from build123d import *

# Parameters (mm, degrees)
BOSS_EXTRUDE1_DEPTH     = 3
SKETCH2_W               = 5
SKETCH2_H               = 3
CUT_EXTRUDE1_DEPTH      = 45.699303997
SKETCH3_W               = 18.054262684
SKETCH3_H               = 80.34146894
BOSS_EXTRUDE2_DEPTH     = 5
SKETCH5_W               = 11.91581337
SKETCH5_H               = 76.008445896
CUT_EXTRUDE2_DEPTH      = 5
CUT_EXTRUDE3_DEPTH      = 45.877920827
CUT_EXTRUDE3_DEPTH_BACK = 45.877920827
SKETCH7_W               = 2
SKETCH7_H               = 9
BOSS_EXTRUDE3_DEPTH     = 5
CUT_EXTRUDE4_DEPTH      = 5
SKETCH9_W               = 2.534423144
SKETCH9_H               = 2
CUT_EXTRUDE5_DEPTH      = 1
CUT_EXTRUDE6_DEPTH      = 2
BOSS_EXTRUDE5_DEPTH     = 2
BOSS_EXTRUDE6_DEPTH     = 2
CUT_EXTRUDE7_START      = -2
CUT_EXTRUDE7_DEPTH      = 2


with BuildPart() as part:
    # Sketch1 → Boss-Extrude1 (new body)
    with BuildSketch(Plane(origin=(0, 0, 0), x_dir=(0, 0, -1), z_dir=(1, 0, 0))):
        with BuildLine():
            Line((-8.833333333, -43), (11.833333333, -43))
            Line((11.833333333, -43), (11.833333333, 43))
            Line((11.833333333, 43), (-8.833333333, 43))
            ThreePointArc((-8.833333333, 43), (-10.954653677, 42.121320344), (-11.833333333, 40))
            Line((-11.833333333, 40), (-11.833333333, -40))
            ThreePointArc((-11.833333333, -40), (-10.954653677, -42.121320344), (-8.833333333, -43))
        make_face()
    extrude(amount=BOSS_EXTRUDE1_DEPTH)

    # Sketch2 → Cut-Extrude1 (cut, through all)
    with BuildSketch(Plane(origin=(3, 0, 0), x_dir=(0, 0, -1), z_dir=(1, 0, 0))):
        with Locations((0, -34.060962647)):
            Rectangle(SKETCH2_W, SKETCH2_H)
    extrude(amount=-CUT_EXTRUDE1_DEPTH, mode=Mode.SUBTRACT)

    # Sketch3 → Boss-Extrude2 (add)
    with BuildSketch(Plane.ZY):
        Rectangle(SKETCH3_W, SKETCH3_H)
    extrude(amount=BOSS_EXTRUDE2_DEPTH)

    # Sketch5 → Cut-Extrude2 (cut)
    with BuildSketch(Plane.ZY.offset(5)):
        Rectangle(SKETCH5_W, SKETCH5_H)
    extrude(amount=-CUT_EXTRUDE2_DEPTH, mode=Mode.SUBTRACT)

    # Sketch6 → Cut-Extrude3 (cut, two sides: drawn at the far end of the back side and taken through both)
    with BuildSketch(Plane.XY.offset(-CUT_EXTRUDE3_DEPTH_BACK)):
        Polygon((-5, -19.974207963), (-1.714874455, -16.689082418), (-1.714874455, 16.689082418), (-5, 19.974207963), align=None)
    extrude(amount=CUT_EXTRUDE3_DEPTH + CUT_EXTRUDE3_DEPTH_BACK, mode=Mode.SUBTRACT)

    # Sketch7 → Boss-Extrude3 (add)
    with BuildSketch(Plane.ZY):
        Rectangle(SKETCH7_W, SKETCH7_H)
    extrude(amount=BOSS_EXTRUDE3_DEPTH)

    # Sketch8 → Cut-Extrude4 (cut)
    with BuildSketch(Plane.XY.offset(1)):
        with BuildLine():
            ThreePointArc((-5, -0.459578833), (-2.44210099, -2.530530169), (0, -0.32421434))
            Line((0, -0.32421434), (0, 0.32421434))
            ThreePointArc((0, 0.32421434), (-2.44210099, 2.530530169), (-5, 0.459578833))
            Line((-5, 0.459578833), (-5, -0.459578833))
        make_face()
        with BuildLine():
            Line((-5, -4.5), (-2.510609776, -4.5))
            ThreePointArc((-2.510609776, -4.5), (-3.81075192, -4.308088951), (-5, -3.748724625))
            Line((-5, -3.748724625), (-5, -4.5))
        make_face()
        with BuildLine():
            Line((-2.510609776, -4.5), (0, -4.5))
            Line((0, -4.5), (0, -3.734546632))
            ThreePointArc((0, -3.734546632), (-1.198256898, -4.304384965), (-2.510609776, -4.5))
        make_face()
        with BuildLine():
            ThreePointArc((-2.510609794, 4.5), (-1.198256907, 4.304384967), (0, 3.734546632))
            Line((0, 3.734546632), (0, 4.5))
            Line((0, 4.5), (-2.510609794, 4.5))
        make_face()
        with BuildLine():
            ThreePointArc((-5, 3.748724625), (-3.810751929, 4.308088948), (-2.510609794, 4.5))
            Line((-2.510609794, 4.5), (-5, 4.5))
            Line((-5, 4.5), (-5, 3.748724625))
        make_face()
    extrude(amount=-CUT_EXTRUDE4_DEPTH, mode=Mode.SUBTRACT)

    # Sketch9 → Cut-Extrude5 (cut)
    with BuildSketch(Plane.ZY.offset(5)):
        Rectangle(SKETCH9_W, SKETCH9_H)
    extrude(amount=-CUT_EXTRUDE5_DEPTH, mode=Mode.SUBTRACT)

    # Sketch12 → Cut-Extrude6 (cut)
    with BuildSketch(Plane.XY.offset(1)):
        with BuildLine():
            Line((-4.836179898, -1), (-5, -1))
            Line((-5, -1), (-5, -3.748724625))
            ThreePointArc((-5, -3.748724625), (-2.497849634, -4.499981909), (0, -3.734546632))
            Line((0, -3.734546632), (0, -0.32421434))
            ThreePointArc((0, -0.32421434), (-2.160279243, -2.507098902), (-4.836179898, -1))
        make_face()
        with BuildLine():
            Line((-5, 3.748724625), (-5, 1))
            Line((-5, 1), (-4.836179898, 1))
            ThreePointArc((-4.836179898, 1), (-2.160279243, 2.507098902), (0, 0.32421434))
            Line((0, 0.32421434), (0, 3.734546632))
            ThreePointArc((0, 3.734546632), (-2.497849634, 4.499981909), (-5, 3.748724625))
        make_face()
    extrude(amount=-CUT_EXTRUDE6_DEPTH, mode=Mode.SUBTRACT)

    # Sketch10 → Boss-Extrude5 (add)
    with BuildSketch(Plane.XY.offset(1)):
        with BuildLine():
            Line((0.632034053, -1.144834058), (-0.193, -4.453864907))
            ThreePointArc((-0.193, -4.453864907), (-2.801828378, -4.592278965), (-5.047908598, -3.258012274))
            Line((-5.047908598, -3.258012274), (-4.41989103, -0.739171385))
            Line((-4.41989103, -0.739171385), (-4.335953587, -0.66680401))
            ThreePointArc((-4.335953587, -0.66680401), (-2.053682052, -3.002243354), (0.632034053, -1.144834058))
        make_face()
        with BuildLine():
            Line((-5.047908598, 3.258012274), (-4.41989103, 0.739171385))
            Line((-4.41989103, 0.739171385), (-4.335953587, 0.66680401))
            ThreePointArc((-4.335953587, 0.66680401), (-2.053682052, 3.002243354), (0.632034053, 1.144834058))
            Line((0.632034053, 1.144834058), (-0.193, 4.453864907))
            ThreePointArc((-0.193, 4.453864907), (-2.801828378, 4.592278965), (-5.047908598, 3.258012274))
        make_face()
    extrude(amount=-BOSS_EXTRUDE5_DEPTH)

    # Sketch13 → Boss-Extrude6 (add)
    with BuildSketch(Plane(origin=(0, 0, -1), x_dir=(-1, 0, 0), z_dir=(0, 0, -1))):
        Polygon((0, 3.679784186), (0.193, 4.453864907), (-0.617433114, 4.244828064), (-0.739085506, -4.079345447), (0.193, -4.453864907), (0, -3.679784186), (0, -2.250971384), (0, 2.250971384), align=None)
    extrude(amount=-BOSS_EXTRUDE6_DEPTH)

    # Sketch15 → Cut-Extrude7 (cut)
    with BuildSketch(Plane(origin=(0, 0, -1), x_dir=(-1, 0, 0), z_dir=(0, 0, -1)).offset(CUT_EXTRUDE7_START)):
        Polygon((4.65583066, 1.685473556), (5.047908598, 3.258012274), (4.038538563, 1.685473556), align=None)
        with BuildLine():
            Line((4.65583066, 1.685473556), (4.038538563, 1.685473556))
            ThreePointArc((4.038538563, 1.685473556), (4.241224486, 1.191898546), (4.335953587, 0.66680401))
            Line((4.335953587, 0.66680401), (4.41989103, 0.739171385))
            Line((4.41989103, 0.739171385), (4.65583066, 1.685473556))
        make_face()
        with BuildLine():
            ThreePointArc((4.335953587, -0.66680401), (4.241224486, -1.191898546), (4.038538563, -1.685473556))
            Line((4.038538563, -1.685473556), (4.65583066, -1.685473556))
            Line((4.65583066, -1.685473556), (4.41989103, -0.739171385))
            Line((4.41989103, -0.739171385), (4.335953587, -0.66680401))
        make_face()
        Polygon((4.65583066, -1.685473556), (4.038538563, -1.685473556), (5.047908598, -3.258012274), align=None)
    extrude(amount=CUT_EXTRUDE7_DEPTH, mode=Mode.SUBTRACT)


solid = part.part
Source: CAD feature listing. Evaluate the final solid. Frame: model axes, mm. A direction names the side the tool comes from. Give positions to 0.01 mm unless a question says otherwise; leave off trailing zeros. Write each loop counter-clockwise with the first axis right and the second up, starting at its lowest first coordinate (ties: lowest second). Pieces come first, ordered by that corner, then holes. Notation, with made-up numbers: (-26, -4.5) -> (2, -4.5) arc R25 ccw to (2, 34.5) -> close; hole circle Ø3 at (24.25, 86). An arc over 180 degrees is marked (long way). Return JSON: item names as keys, results as strings. Group by question number.
1. Section B-B, the plane y = 10.5. Output: boundary loops of the cut face in (x, z).
2. Pin query (flat end, axial travel): pin 1 Ø10 at (y, z) = (10.5, -1) entering from -X; pin 2 Ø2.5 at (x, y) = (-3.5, -15) entering from -Z; pin 3 Ø5 at (y, z) = (-17, -9) entering from -X; pin 4 Ø1.5 at (x, z) = (-2.5, -1.5) entering from -Y. Return the tip coordinate at first contact, or that it passes through.
3. Section A-A, the plane z = 1.75. Output: boundary loops of the cut face in (x, y), then the cut area to 3 significant figures.
4. Section C-C, the plane x = -3. Output: boundary loops of the cut face in (y, z), then the cut area to 3 significant figures.
5. Mould query, pull axis Z, two halves, no side actions, for faces 1 (the face through (-1.715, 0, -8)), 2 (the face through (1.479, -42.098, 10.978)), 3 (the face through (-2.195, 2.985, 0.014)). Classes: +Z half, -Z half, draft (parallel to the pull), parting line (faces both ways), or undercut.
6. Access query for faces 4 (the face through (-3, 38.004, 0)), 5 (the face through (-3.334, 18.309, 7.471)), 6 (the face through (-2, -40.171, 0)). Directions: +Z, -Z, +X, -X, +Y, -Y. A direction counts if a zero-diameter tool reaches every point of the face in a straight line with its end or side. Return the directions, or none.
7. Material intervals for line 1 (Y direction, x = -1.75, z = -2.75); line 2 (Z direction, x = -2.5, y = 34); line 3 (X direction, y = 1, z = -6), sorted ascending. Write a range as from..to.
8. Section D-D, the plane z = -8.25. Output: boundary loops of the cut face in (x, y).
Determined:
{
 "1": {"outline": "(-1.71, -9.03) -> (0, -9.03) -> (0, -11.83) -> (3, -11.83) -> (3, 11.83) -> (0, 11.83) -> (0, 9.03) -> (-1.71, 9.03) -> (-1.71, 5.96) -> (0, 5.96) -> (0, -5.96) -> (-1.71, -5.96) -> close"},
 "2": {"pin 1": "stops at x = -1.71", "pin 2": "passes through", "pin 3": "stops at x = -4.53", "pin 4": "stops at y = -40.17"},
 "3": {"outline": "(-5, -40.17) -> (0, -40.17) -> (0, -43) -> (3, -43) -> (3, -35.56) -> (0, -35.56) -> (0, -38) -> (-5, -38) -> close; (-5, 38) -> (0, 38) -> (0, -32.56) -> (3, -32.56) -> (3, 43) -> (0, 43) -> (0, 40.17) -> (-5, 40.17) -> close", "area": "271 mm2"},
 "4": {"outline": "(-40.17, -9.03) -> (-17.97, -9.03) -> (-17.97, -5.96) -> (-38, -5.96) -> (-38, 5.96) -> (-17.97, 5.96) -> (-17.97, 9.03) -> (-40.17, 9.03) -> close; (-4.54, -1) -> (-2.72, -1) -> (-2.72, 1) -> (-4.54, 1) -> close; (2.72, -1) -> (4.54, -1) -> (4.54, 1) -> (2.72, 1) -> close; (17.97, -9.03) -> (40.17, -9.03) -> (40.17, 9.03) -> (17.97, 9.03) -> (17.97, 5.96) -> (38, 5.96) -> (38, -5.96) -> (17.97, -5.96) -> close", "area": "331 mm2"},
 "5": {"face 1": "draft", "face 2": "+Z half", "face 3": "undercut"},
 "6": {"face 4": "-X", "face 5": "+Z, -Z, -X", "face 6": "+Z, -Z, -X, -Y"},
 "7": {"line 1": "y = -40.17..-38, 38..40.17", "line 2": "z = -9.03..-5.96, 5.96..9.03", "line 3": "x = -1.71..3"},
 "8": {"outline": "(-5, -40.17) -> (0, -40.17) -> (0, -43) -> (3, -43) -> (3, 43) -> (0, 43) -> (0, 40.17) -> (-5, 40.17) -> (-5, 19.97) -> (-1.71, 16.69) -> (-1.71, -16.69) -> (-5, -19.97) -> close"}
}
